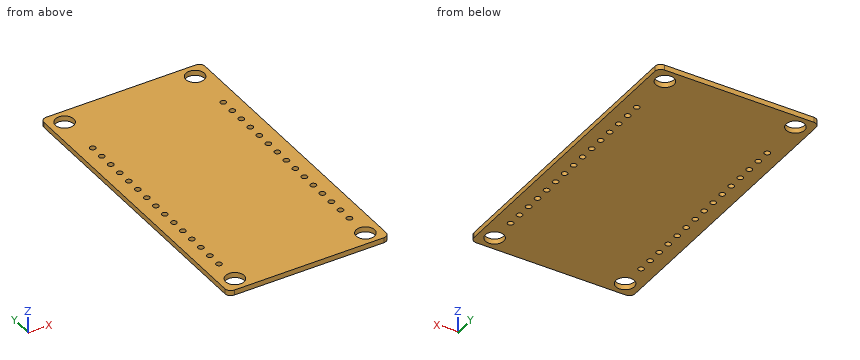
```python
from build123d import *

# Parameters (mm, degrees)
ESBO_O1_W                = 28
ESBO_O1_H                = 53
RESSALTO_EXTRUS_O1_DEPTH = 0.45
CORTE_EXTRUS_O1_REACH    = 31.984
ESBO_O4_R                = 1.6
CORTE_EXTRUS_O2_REACH    = 31.984
ESBO_O5_R                = 0.5
PADR_O_LINEAR1_COUNT     = 15
PADR_O_LINEAR1_PITCH     = 2.54
FILETE1_R                = 1


with BuildPart() as part:
    # Esbo_o1 → Ressalto-extrus_o1 (new, symmetric)
    with BuildSketch(Plane.XY):
        Rectangle(ESBO_O1_W, ESBO_O1_H)
    extrude(amount=RESSALTO_EXTRUS_O1_DEPTH, both=True)

    # Esbo_o4 → Corte-extrus_o1 (cut, up to next)
    with BuildSketch(Plane.XY.offset(0.45), mode=Mode.PRIVATE) as corte_extrus_o1_sk1:
        with Locations((-11.35, -24)):
            Circle(ESBO_O4_R)
    corte_extrus_o1_tool1 = extrude(corte_extrus_o1_sk1.sketch, amount=-CORTE_EXTRUS_O1_REACH, mode=Mode.PRIVATE) & part.part
    # Esbo_o4 → Corte-extrus_o1 (cut, up to next)
    with BuildSketch(Plane.XY.offset(0.45), mode=Mode.PRIVATE) as corte_extrus_o1_sk2:
        with Locations((11.35, -24)):
            Circle(ESBO_O4_R)
    corte_extrus_o1_tool2 = extrude(corte_extrus_o1_sk2.sketch, amount=-CORTE_EXTRUS_O1_REACH, mode=Mode.PRIVATE) & part.part
    # Esbo_o4 → Corte-extrus_o1 (cut, up to next)
    with BuildSketch(Plane.XY.offset(0.45), mode=Mode.PRIVATE) as corte_extrus_o1_sk3:
        with Locations((11.35, 24)):
            Circle(ESBO_O4_R)
    corte_extrus_o1_tool3 = extrude(corte_extrus_o1_sk3.sketch, amount=-CORTE_EXTRUS_O1_REACH, mode=Mode.PRIVATE) & part.part
    # Esbo_o4 → Corte-extrus_o1 (cut, up to next)
    with BuildSketch(Plane.XY.offset(0.45), mode=Mode.PRIVATE) as corte_extrus_o1_sk4:
        with Locations((-11.35, 24)):
            Circle(ESBO_O4_R)
    corte_extrus_o1_tool4 = extrude(corte_extrus_o1_sk4.sketch, amount=-CORTE_EXTRUS_O1_REACH, mode=Mode.PRIVATE) & part.part
    add(corte_extrus_o1_tool1.solids().sort_by_distance((-11.35, -24, 0.45))[0], mode=Mode.SUBTRACT)
    add(corte_extrus_o1_tool2.solids().sort_by_distance((11.35, -24, 0.45))[0], mode=Mode.SUBTRACT)
    add(corte_extrus_o1_tool3.solids().sort_by_distance((11.35, 24, 0.45))[0], mode=Mode.SUBTRACT)
    add(corte_extrus_o1_tool4.solids().sort_by_distance((-11.35, 24, 0.45))[0], mode=Mode.SUBTRACT)

    # Esbo_o5 → Corte-extrus_o2 (cut, up to next)
    with BuildSketch(Plane.XY.offset(0.45), mode=Mode.PRIVATE) as corte_extrus_o2_sk1:
        with Locations((-11.35, -19.5)):
            Circle(ESBO_O5_R)
    corte_extrus_o2_tool1 = extrude(corte_extrus_o2_sk1.sketch, amount=-CORTE_EXTRUS_O2_REACH, mode=Mode.PRIVATE) & part.part
    # Esbo_o5 → Corte-extrus_o2 (cut, up to next)
    with BuildSketch(Plane.XY.offset(0.45), mode=Mode.PRIVATE) as corte_extrus_o2_sk2:
        with Locations((11.35, -19.5)):
            Circle(ESBO_O5_R)
    corte_extrus_o2_tool2 = extrude(corte_extrus_o2_sk2.sketch, amount=-CORTE_EXTRUS_O2_REACH, mode=Mode.PRIVATE) & part.part
    corte_extrus_o2_1 = corte_extrus_o2_tool1.solids().sort_by_distance((-11.35, -19.5, 0.45))[0]
    add(corte_extrus_o2_1, mode=Mode.SUBTRACT)
    corte_extrus_o2_2 = corte_extrus_o2_tool2.solids().sort_by_distance((11.35, -19.5, 0.45))[0]
    add(corte_extrus_o2_2, mode=Mode.SUBTRACT)
    corte_extrus_o2 = corte_extrus_o2_1 + corte_extrus_o2_2  # Corte-extrus_o2 as one shape, for the pattern or mirror that repeats it

    # Padr_o linear1: Corte-extrus_o2 ×15
    with Locations(*[(0, i * PADR_O_LINEAR1_PITCH, 0) for i in range(1, PADR_O_LINEAR1_COUNT)]):
        add(corte_extrus_o2, mode=Mode.SUBTRACT)

    # Filete1
    filete1_edges = [part.edges().sort_by_distance(p)[0] for p in [
        (-14, 26.5, 0),
        (14, 26.5, 0),
        (14, -26.5, 0),
        (-14, -26.5, 0),
    ]]
    fillet(filete1_edges, radius=FILETE1_R)


solid = part.part
```
The model under review builds one solid part; all positions refer to its coordinate system, in mm. Round coordinates to 2 decimals unless told otherwise and drop trailing zeros. Loops run counter-clockwise (first coordinate to the right, second up) from the corner with the lowest first, then second, coordinate; pieces in that order, holes last. Notation, with made-up numbers: (-6.5, -24) - (42.5, -24) arc R30 ccw to (42.5, 6) - close; hole circle Ø2 at (67.25, 49). An arc over 180 degrees is marked (long way). Use a Markdown table: item, result. Add a question column.
Q1. For probe 1 along Y at (x, z) = (-10, -0.3); probe 2 along X at (y, z) = (3.5, -0.3), list the stretches that pass through material, from the lowest coordinate up.
Q2. Add section C-C (x = -11.35). State how many separate pieces and enclosed holes the cut face has, plus the area to 3 significant figures.
Q3. Add section A-A (y = 16.06). State the section outline as (x, z) points.
Q4. Insertion check: pin 1 Ø1.9 at (x, y) = (-11.35, -24) entering from -Z. The pin has a flat end and moves straight along its axis. Give the tip position at first contact, or say it passes through.
Q5. Add section B-B (y = 24). State the section outline as (x, z) points.
Worked answers:
| question | item | result |
|---|---|---|
| 1 | probe 1 | -26.5 to -24.86, -23.14 to 23.14, 24.86 to 26.5 |
| 1 | probe 2 | -14 to -11.83, -10.87 to 10.87, 11.83 to 14 |
| 2 | separate pieces | 18 |
| 2 | enclosed holes | 0 |
| 2 | area | 28.4 mm² |
| 3 | outline | (-14, -0.45) - (-11.85, -0.45) - (-11.85, 0.45) - (-14, 0.45) - close; (-10.85, -0.45) - (10.85, -0.45) - (10.85, 0.45) - (-10.85, 0.45) - close; (11.85, -0.45) - (14, -0.45) - (14, 0.45) - (11.85, 0.45) - close |
| 4 | pin 1 | through |
| 5 | outline | (-14, -0.45) - (-12.95, -0.45) - (-12.95, 0.45) - (-14, 0.45) - close; (-9.75, -0.45) - (9.75, -0.45) - (9.75, 0.45) - (-9.75, 0.45) - close; (12.95, -0.45) - (14, -0.45) - (14, 0.45) - (12.95, 0.45) - close |
